from build123d import *

# Parameters (mm, degrees)
F2_W     = 8
F2_H     = 1.5
F3_DEPTH = 6.63


with BuildPart() as f1:
    # F0 (on Right) → F1 (revolve)
    with BuildSketch(Plane.YZ):
        Polygon((2, 8.8), (2, 0), (3, 0), (3, 8), (3.5, 8), (3.5, 8.8), align=None)
    revolve(axis=Axis((0, 0, 4.285715), (0, 0, 1)))

    # F2 (on face) → F3 (cut)
    with BuildSketch(Plane(origin=(0, 0, 0), x_dir=(1, 0, 0), z_dir=(0, 0, -1))):
        Rectangle(F2_W, F2_H)
    extrude(amount=-F3_DEPTH, mode=Mode.SUBTRACT)


solid = f1.part
Geometry: final body of the model. Coordinates: model frame, mm. A direction names the side the tool comes from. Give positions to 0.01 mm unless a question says otherwise; leave off trailing zeros. Loops run counter-clockwise (first coordinate to the right, second up) from the corner with the lowest first, then second, coordinate; pieces in that order, holes last. Notation, with made-up numbers: (-23.75, 40.5) - (2.25, 40.5) arc R38 ccw to (2.25, 78.5) - close; hole circle Ø1 at (42.5, 10). An arc over 180 degrees is marked (long way). One line per question, with ' | ' between items. Start each with the question number.
(1) Ray query, line 1 (X direction, y = 0, z = 6.75); line 2 (Y direction, x = -2, z = 2.25). Return the intervals inside material, ascending. Write a range as from..to.
(2) Contact query for flat-ended pins moving along their axis: pin 1 (2 mm diameter, centred on y = 0, z = 5, fed in from +X); pin 2 (0.8 mm diameter, centred on x = -2.5, z = 2.5, fed in from -Y); pin 3 (3 mm diameter, centred on y = -1, z = 4, fed in from -X). Output: stop coordinate, or through.
(3) Section query B-B on y = 0. Return loops of the section in (x, z), then the cut area to 3 significant figures.
(4) Pull-direction query (Y, two-part tool) for faces 1 (the flat face through (0, -2.4, 0)), 2 (the flat face through (2.4, 0, 6.63)), 3 (the cylindrical face through (1.15, 2.77, 4.06)); classes: released by +Y, released by -Y, zero draft, split by the parting line, or undercut.
(5) Section query D-D on x = 2.75. Return loops of the section in (y, z), then the cut area to 3 significant figures.
(6) Section query A-A on z = 4. Return loops of the section in (x, y).
(7) Reachability of faces 4 (the cylindrical face through (0.766, 1.847, 4.338)), 5 (the flat face through (2.4, -0.75, 3.3)), 6 (the flat face through (-1, -3, 8)) from +Z, -Z, +X, -X, +Y, -Y: full face, straight path, thin tool, end or side. Return the list, or none.
(8) Section query C-C on x = 0. Return loops of the section in (y, z), then the cut area to 3 significant figures.
The answers:
1) line 1: -3..-2, 2..3 | line 2: -2.24..-0.75, 0.75..2.24
2) pin 1: x = 2.9 | pin 2: y = -2.14 | pin 3: x = -2.9
3) outline: (-3.5, 8) - (-3, 8) - (-3, 6.63) - (-2, 6.63) - (-2, 8.8) - (-3.5, 8.8) - close; (2, 6.63) - (3, 6.63) - (3, 8) - (3.5, 8) - (3.5, 8.8) - (2, 8.8) - close | area: 5.14 mm2
4) face 1: zero draft | face 2: undercut | face 3: split by the parting line
5) outline: (-2.17, 8) - (-1.2, 8) - (-1.2, 0) - (-0.75, 0) - (-0.75, 6.63) - (0.75, 6.63) - (0.75, 0) - (1.2, 0) - (1.2, 8) - (2.17, 8) - (2.17, 8.8) - (-2.17, 8.8) - close | area: 12.7 mm2
6) outline: (-2.9, -0.75) arc R3 ccw to (2.9, -0.75) - (1.85, -0.75) arc R2 cw to (-1.85, -0.75) - close; (-2.9, 0.75) - (-1.85, 0.75) arc R2 cw to (1.85, 0.75) - (2.9, 0.75) arc R3 ccw to start
7) face 4: +Z, -Z | face 5: -Z, +X, -X | face 6: -Z
8) outline: (-3.5, 8) - (-3, 8) - (-3, 0) - (-2, 0) - (-2, 8.8) - (-3.5, 8.8) - close; (2, 0) - (3, 0) - (3, 8) - (3.5, 8) - (3.5, 8.8) - (2, 8.8) - close | area: 18.4 mm2
